```python
from build123d import *

# Parameters (mm, degrees)
SKETCH045_W     = 80
SKETCH045_H     = 42
PAD009_DEPTH    = 5
SKETCH047_R     = 12
SKETCH047_R_2   = 1.75
POCKET022_DEPTH = 5
SKETCH049_R     = 3.474866
SKETCH049_R_2   = 3.27743
POCKET025_DEPTH = 2


with BuildPart() as part:
    # Sketch045 → Pad009 (new body)
    with BuildSketch(Plane.XY):
        with Locations((0, 11)):
            Rectangle(SKETCH045_W, SKETCH045_H)
    extrude(amount=PAD009_DEPTH)

    # Sketch047 (on Face5 of Pad009) → Pocket022 (cut)
    with BuildSketch(Plane(origin=(0, 0, 0), x_dir=(1, 0, 0), z_dir=(0, 0, -1))):
        with Locations((8, -9)):
            Circle(SKETCH047_R)
        with Locations((-7.5, 6.5)):
            Circle(SKETCH047_R_2)
        with Locations((23.5, 6.5)):
            Circle(SKETCH047_R_2)
        with Locations((-7.5, -24.5)):
            Circle(SKETCH047_R_2)
        with Locations((23.5, -24.5)):
            Circle(SKETCH047_R_2)
        with BuildLine():
            ThreePointArc((-28.25, -11), (-30, -9.25), (-31.75, -11))
            Line((-31.75, -11), (-31.75, -15))
            ThreePointArc((-31.75, -15), (-30, -16.75), (-28.25, -15))
            Line((-28.25, -11), (-28.25, -15))
        make_face()
        with BuildLine():
            ThreePointArc((31.75, -11), (30, -9.25), (28.25, -11))
            Line((28.25, -11), (28.25, -15))
            ThreePointArc((28.25, -15), (30, -16.75), (31.75, -15))
            Line((31.75, -11), (31.75, -15))
        make_face()
    extrude(amount=-POCKET022_DEPTH, mode=Mode.SUBTRACT)

    # Sketch049 (on Face5 of Pocket022) → Pocket025 (cut)
    with BuildSketch(Plane.XY.offset(5)):
        with Locations((-7.509294, 24.561527)):
            Circle(SKETCH049_R)
        with Locations((23.476507, 24.473993)):
            Circle(SKETCH049_R_2)
    extrude(amount=-POCKET025_DEPTH, mode=Mode.SUBTRACT)


with BuildPart() as part_1:
    # Body004 placement: moved
    add(part.part.moved(Location((0, 0, -5))))


solid = part_1.part
```
Here's how the part is built. I have some questions about the finished solid (model axes, mm). A direction names the side the tool comes from. Round coordinates to 2 decimals unless told otherwise and drop trailing zeros. Order: outer loops, then holes, each group sorted by start corner. A loop starts at its lowest first (then second) coordinate and runs counter-clockwise, first axis right, second up. Notation, with made-up numbers: M 11.5,-26 L 59.5,-26 A27 ccw 59.5,5 Z; hole C 30.25,65.25 d9. An arc over 180 degrees is marked long. Use CSV: the item, a comma, the result in double quotes.
1) I want a section at A-A (z = -3.9). List the corners of the cut face in (x, y) for me, then the cut area to 3 significant figures.
Taken from the geometry:
outline,"M -40,-10 L 40,-10 L 40,32 L -40,32 Z; hole M -31.75,11 A1.75 ccw -28.25,11 L -28.25,15 A1.75 ccw -31.75,15 Z; hole C -7.5,-6.5 d3.5; hole C -7.5,24.5 d3.5; hole C 8,9 d24; hole C 23.5,-6.5 d3.5; hole C 23.5,24.5 d3.5; hole M 28.25,11 A1.75 ccw 31.75,11 L 31.75,15 A1.75 ccw 28.25,15 Z"
area,"2,820 mm^2"
2) I want a section at D-D (x = -7.5). List the corners of the cut face in (y, z) for me, then the cut area to 3 significant figures.
Taken from the geometry:
outline,"M -10,-5 L -8.25,-5 L -8.25,0 L -10,0 Z; M -4.75,-5 L 22.75,-5 L 22.75,-2 L 21.09,-2 L 21.09,0 L -4.75,0 Z; M 26.25,-5 L 32,-5 L 32,0 L 28.04,0 L 28.04,-2 L 26.25,-2 Z"
area,"168 mm^2"
3) I'm going to push flat-ended pins straight in: P1, Ø7.5, axis at x = 23.48, y = 24.47, coming from the +Z side; P2, Ø2, axis at x = 24, y = 23, coming from the +Z side. Where does each tip first touch, or does it pass through?
Taken from the geometry:
P1,"z = 0"
P2,"z = -2"
4) I want a section at C-C (y = -6.5). List the corners of the cut face in (x, z) for me, then the cut area to 3 significant figures.
Taken from the geometry:
outline,"M -40,-5 L -9.25,-5 L -9.25,0 L -40,0 Z; M -5.75,-5 L 21.75,-5 L 21.75,0 L -5.75,0 Z; M 25.25,-5 L 40,-5 L 40,0 L 25.25,0 Z"
area,"365 mm^2"
5) On a 3-axis mill with a long thin cutter (end or side, diameter ignored), from which of +Z, -Z, +X, -X, +Y, -Y can I reach the whole of each face in a straight line? I mean faces 1 (the flat face through (-6, 23, -2)), 2 (the flat face through (-9, 11, -5)), 3 (the flat face through (-28.25, 13, -3)). Say none if no direction works.
Taken from the geometry:
face 1,"+Z"
face 2,"-Z, +X, -X, +Y, -Y"
face 3,"+Z, -Z"
6) I want a section at B-B (x = 8). List the corners of the cut face in (y, z) for me, then the cut area to 3 significant figures.
Taken from the geometry:
outline,"M -10,-5 L -3,-5 L -3,0 L -10,0 Z; M 21,-5 L 32,-5 L 32,0 L 21,0 Z"
area,"90.0 mm^2"
7) I need wall thicknesses on line 1 along Y through (x, z) = (-7.5, -0.95); line 2 along Y through (x, z) = (23.5, -2.65); line 3 along X through (y, z) = (-6.5, -1.6). Which ranges of each line are inside material? Lowest first, please. Write a range as [from, to].
Taken from the geometry:
line 1,"[-10, -8.25], [-4.75, 21.09], [28.04, 32]"
line 2,"[-10, -8.25], [-4.75, 22.75], [26.25, 32]"
line 3,"[-40, -9.25], [-5.75, 21.75], [25.25, 40]"
